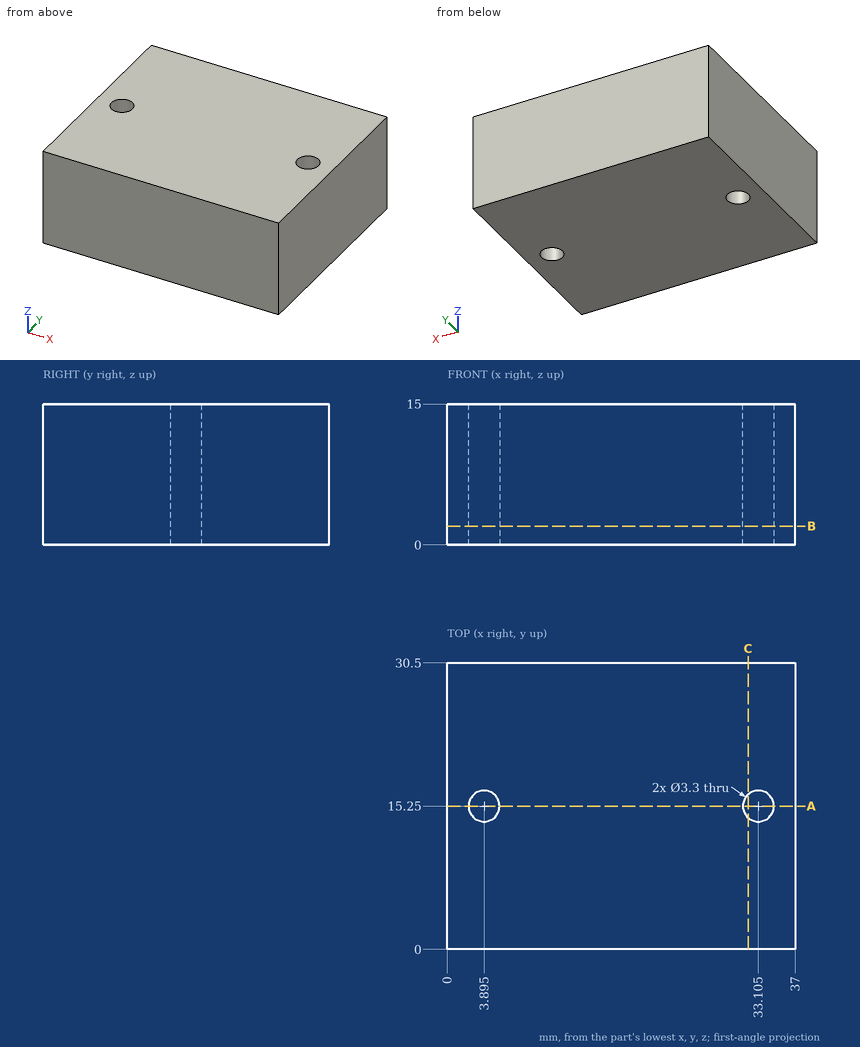
Can you work these out from the drawing? Everything is in mm from the part's minimum corner. Round coordinates to 2 decimals unless told otherwise and drop trailing zeros. Write each loop counter-clockwise with the first axis right and the second up, starting at its lowest first coordinate (ties: lowest second). Pieces come first, ordered by that corner, then holes. Notation, with made-up numbers: (-27, -2.75) - (-2, -2.75) arc R35 ccw to (-2, 29.25) - close; hole circle Ø3 at (67, -33.75). An arc over 180 degrees is marked (long way). Use a Markdown table: item, result.
Q1. Please list where this line runs through material, in increasing order: L1, parallel to Y at x = 5, z = 1.25.
Output values:
| item | result |
|---|---|
| L1 | 0 to 14.02, 16.48 to 30.5 |
Q2. I want a section at C-C (x = 32). List the corners of the cut face in (y, z) for me, plus the area to 3 significant figures.
Output values:
| item | result |
|---|---|
| outline | (0, 0) - (14.02, 0) - (14.02, 15) - (0, 15) - close; (16.48, 0) - (30.5, 0) - (30.5, 15) - (16.48, 15) - close |
| area | 421 mm2 |
Q3. I want a section at B-B (z = 2). List the corners of the cut face in (x, y) for me (3 decimals).
Output values:
| item | result |
|---|---|
| outline | (0, 0) - (37, 0) - (37, 30.5) - (0, 30.5) - close; hole circle Ø3.3 at (3.895, 15.25); hole circle Ø3.3 at (33.105, 15.25) |
Q4. I want a section at A-A (y = 15.25). List the corners of the cut face in (x, z) for me (3 decimals).
Output values:
| item | result |
|---|---|
| outline | (0, 0) - (2.245, 0) - (2.245, 15) - (0, 15) - close; (5.545, 0) - (31.455, 0) - (31.455, 15) - (5.545, 15) - close; (34.755, 0) - (37, 0) - (37, 15) - (34.755, 15) - close |
